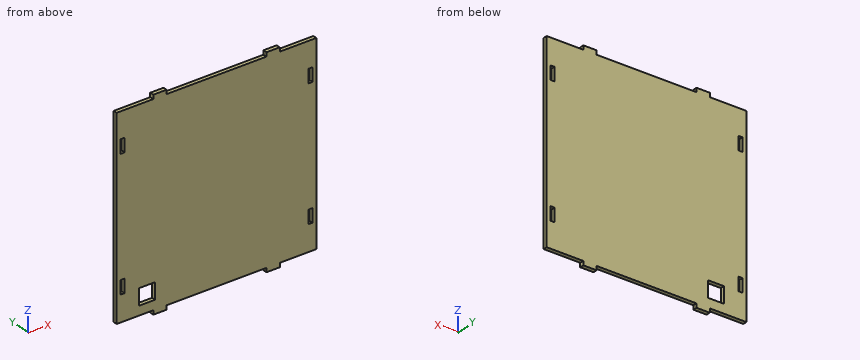
```python
from build123d import *

# Parameters (mm, degrees)
F0_W     = 12
F0_H     = 12
F0_W_2   = 2.98
F0_H_2   = 10
F1_DEPTH = 3


with BuildPart() as f1:
    # F0 (on Front) → F1 (new body)
    with BuildSketch(Plane.XZ):
        Polygon((-47.500234, 72), (-75.000234, 72), (-74.999766, -72), (-47.499766, -72), (-47.499766, -75), (-37.499766, -75), (-37.499766, -72), (37.500234, -72), (37.500234, -75), (47.500234, -75), (47.500234, -72), (75.000234, -72), (74.999766, 72), (47.5, 72), (47.5, 75), (37.5, 75), (37.5, 72.005854), (-37.5, 72), (-37.500234, 75), (-47.500234, 75), align=None)
        with Locations((-52.06838, -59.269677)):
            Rectangle(F0_W, F0_H, mode=Mode.SUBTRACT)
        with Locations((-70.510156, -48)):
            Rectangle(F0_W_2, F0_H_2, mode=Mode.SUBTRACT)
        with Locations((70.510156, -48)):
            Rectangle(F0_W_2, F0_H_2, mode=Mode.SUBTRACT)
        with Locations((-70.510156, 48)):
            Rectangle(F0_W_2, F0_H_2, mode=Mode.SUBTRACT)
        with Locations((70.510156, 48)):
            Rectangle(F0_W_2, F0_H_2, mode=Mode.SUBTRACT)
    extrude(amount=F1_DEPTH)


solid = f1.part
```
Read the model definition and answer for the solid it produces. Units are mm, in the model's axes. Round coordinates to 2 decimals unless told otherwise and drop trailing zeros. Write each loop counter-clockwise with the first axis right and the second up, starting at its lowest first coordinate (ties: lowest second). Pieces come first, ordered by that corner, then holes. Notation, with made-up numbers: (-15, 84) - (37, 84) arc R22 cw to (37, 93) - close; hole circle Ø8 at (26.5, -26.5). An arc over 180 degrees is marked (long way). Use CSV: the item, a comma, the result in double quotes.
Q1. Find section A-A, the plane x = -54. Write down the section's boundary in (y, z), then the cut area to 3 significant figures.
Values:
outline,"(-3, -72) - (0, -72) - (0, -65.27) - (-3, -65.27) - close; (-3, -53.27) - (0, -53.27) - (0, 72) - (-3, 72) - close"
area,"396 mm²"
Q2. Each of these flat-tipped pins is pushed along its axis until it touches: pin 1 Ø0.9 at (x, y) = (70, -1) entering from +Z; pin 2 Ø1.5 at (y, z) = (-2, -74) entering from +X. Where does it stop, or does it pass through?
Values:
pin 1,"stops at z = 72"
pin 2,"stops at x = 47.5"
Q3. Find section C-C, the plane x = 60. Write down the section's boundary in (y, z).
Values:
outline,"(-3, -72) - (0, -72) - (0, 72) - (-3, 72) - close"
Q4. Straight lines are drawn through the part: line 1 along X through (y, z) = (-1.2, 47); line 2 along Z through (x, y) = (-57, -1); line 3 along X through (y, z) = (-1.65, -54). For each, find the intervals that lie inside material, in ascending order.
Values:
line 1,"x = -75 to -72, -69.02 to 69.02, 72 to 75"
line 2,"z = -72 to -65.27, -53.27 to 72"
line 3,"x = -75 to -58.07, -46.07 to 75"
Q5. Find section B-B, the plane y = -0.9. Count the separate pieces of the cut face and the enclosed holes in it, then the cut area to 3 significant figures.
Values:
separate pieces,"1"
enclosed holes,"5"
area,"21,500 mm²"
